The figure shows three views and two pictorial views of one solid part (mm, origin at its lowest corner). Answer the questions. A direction names the side the tool comes from. Give positions to 0.01 mm unless a question says otherwise; leave off trailing zeros. Loops run counter-clockwise (first coordinate to the right, second up) from the corner with the lowest first, then second, coordinate; pieces in that order, holes last. Notation, with made-up numbers: M 66.25,73.25 L 75.25,73.25 A17 ccw 75.25,86.25 Z; hole C 37.5,79.5 d7. An arc over 180 degrees is marked long. Answer as a JSON object with one key per item and string values. Group by question number.
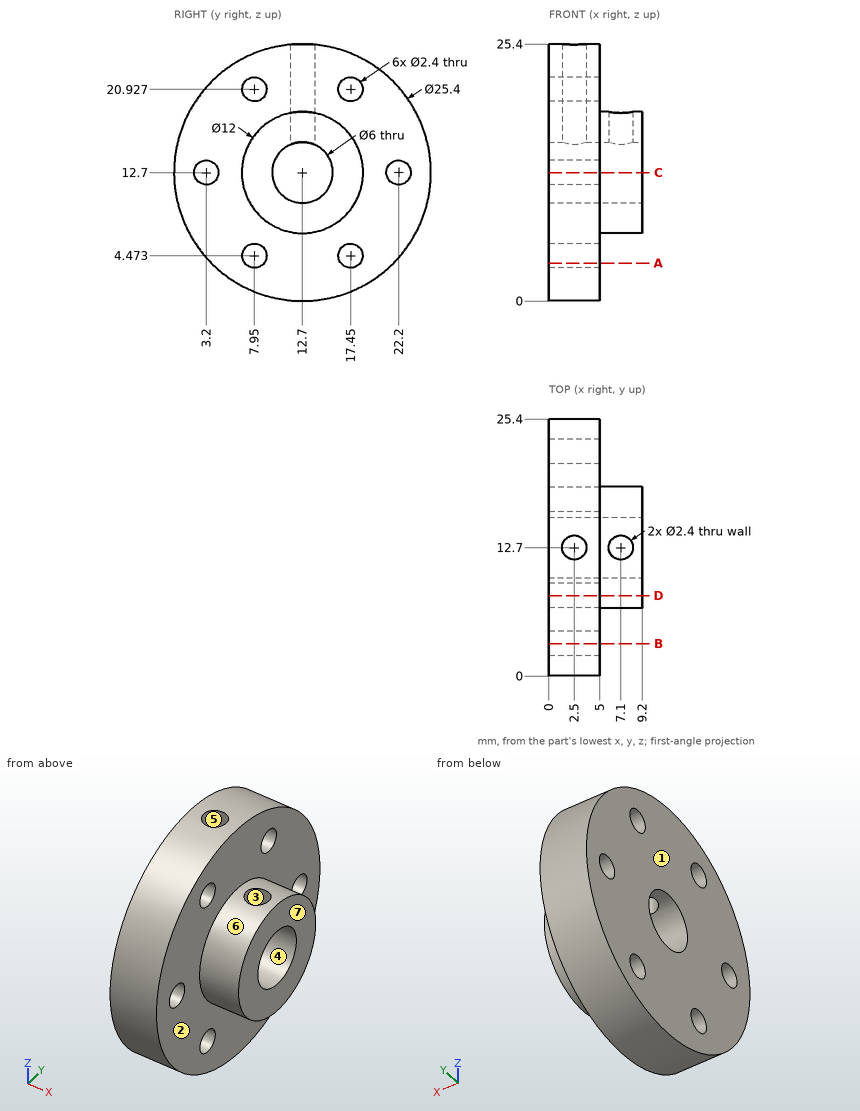
Item 1: Find the intervals of material crossed by probe 1 along Z at (x, y) = (2.25, 7.95); probe 2 along X at (y, z) = (21, 7.25); probe 3 along Z at (x, y) = (1.25, 22.2), in increasing order. Write a range as [from, to].
Item 2: For a pull along Y with two mould halves and no side action, classify the marked faces 4, 5, 6 and 7 as pulls with the +Y half, pulls with the -Y half, needs draft (parallel to the pull), parting line crosses it, or undercut.
Item 3: A tool of negligible diameter and unlimited length cuts with its end or side. For the marked faces 1, 2 and 3, from which of +Z, -Z, +X, -X, +Y, -Y can it reach the whole face along a straight path? Write none if from no direction.
Item 4: A cutting plane is placed at B-B (y = 3.2). Determine the outline of the cut face in (x, z), and give its area (3 significant figures).
Item 5: A cutting plane is placed at D-D (y = 7.95). Determine the outline of the cut face in (x, z), and give its area (3 significant figures).
Item 6: A cutting plane is placed at C-C (z = 12.7). Determine the outline of the cut face in (x, y), and give its area (3 significant figures).
Item 7: Given pin 1 Ø3 at (x, y) = (8, 8.5) entering from +Z; pin 2 Ø2 at (y, z) = (7.95, 20.93) entering from +X; pin 3 Ø3 at (y, z) = (3.2, 12.7) entering from +X; pin 4 Ø1 at (x, z) = (7, 13.5) entering from -Y, each flat-ended and moving along its own axis, determine where each tip first touches the part or whether it passes through.
Item 8: A cutting plane is placed at A-A (z = 3.75). Determine the outline of the cut face in (x, y).
The answers:
{
 "1": {"probe 1": "z = [0.92, 3.27], [5.67, 19.73], [22.13, 24.48]", "probe 2": "x = [0, 5]", "probe 3": "z = [4.27, 11.5], [13.9, 21.13]"},
 "2": {"face 4": "undercut", "face 5": "undercut", "face 6": "parting line crosses it", "face 7": "needs draft"},
 "3": {"face 1": "+Z, -Z, -X, +Y, -Y", "face 2": "+X", "face 3": "+Z"},
 "4": {"outline": "M 0,4.27 L 5,4.27 L 5,11.5 L 0,11.5 Z; M 0,13.9 L 5,13.9 L 5,21.13 L 0,21.13 Z", "area": "72.3 mm^2"},
 "5": {"outline": "M 0,0.92 L 5,0.92 L 5,3.27 L 0,3.27 Z; M 0,5.67 L 5,5.67 L 5,9.03 L 9.2,9.03 L 9.2,16.37 L 5,16.37 L 5,19.73 L 0,19.73 Z; M 0,22.13 L 5,22.13 L 5,24.48 L 0,24.48 Z", "area": "125 mm^2"},
 "6": {"outline": "M 0,0 L 5,0 L 5,2 L 0,2 Z; M 0,4.4 L 5,4.4 L 5,6.7 L 9.2,6.7 L 9.2,9.7 L 0,9.7 Z; M 0,15.7 L 9.2,15.7 L 9.2,18.7 L 5,18.7 L 5,21 L 0,21 Z; M 0,23.4 L 5,23.4 L 5,25.4 L 0,25.4 Z", "area": "98.2 mm^2"},
 "7": {"pin 1": "stops at z = 18.06", "pin 2": "passes through", "pin 3": "stops at x = 5", "pin 4": "stops at y = 6.71"},
 "8": {"outline": "M 0,3.69 L 5,3.69 L 5,6.99 L 0,6.99 Z; M 0,8.91 L 5,8.91 L 5,16.49 L 0,16.49 Z; M 0,18.41 L 5,18.41 L 5,21.71 L 0,21.71 Z"}
}
